Geometry: final body of the model. Coordinates: model frame, mm. A direction names the side the tool comes from. Give positions to 0.01 mm unless a question says otherwise; leave off trailing zeros. Write each loop counter-clockwise with the first axis right and the second up, starting at its lowest first coordinate (ties: lowest second). Pieces come first, ordered by that corner, then holes. Notation, with made-up numbers: M 29.5,65 L 72.5,65 A29 cw 72.5,91 Z; hole C -37,85.5 d11. An arc over 180 degrees is marked long. Use one line per item in the form item = value. Start each with the question number.
Item 1: Section query B-B on y = -25.5. Return loops of the section in (x, z).
Item 2: Access query for faces 1 (the flat face through (-27, -28.875, 12)), 2 (the flat face through (-41.999, -28, 12)). Directions: +Z, -Z, +X, -X, +Y, -Y. A direction counts if a zero-diameter tool reaches every point of the face in a straight line with its end or side. Return the directions, or none.
Item 3: Section query A-A on z = 10.75. Return loops of the section in (x, y), then the cut area to 3 significant figures.
Item 4: Contact query for flat-ended pins moving along their axis: P1, Ø2, axis at y = -27, z = 9, coming from the +X side; P2, Ø4.5, axis at x = -29, z = 10, coming from the +Y side; P3, Ø1, axis at x = -37.5, z = 7.5, coming from the -Y side (3 decimals). Output: stop coordinate, or through.
Item 5: Section query C-C on x = -30.5. Return loops of the section in (y, z).
Item 6: Material intervals for line 1 along X through (y, z) = (-26.75, 6.5); line 2 along Y through (x, z) = (-31.75, 10.75); line 3 along Y through (x, z) = (-25.25, 12), sorted ascending. Write a range as from..to.
from build123d import *

# Parameters (mm, degrees)
F1_DEPTH = 25


with BuildPart() as f1:
    # F0 (on Top) → F1 (new body)
    with BuildSketch(Plane.XY):
        Polygon((-32.0135473862, -18.9185493521), (-41.9985689223, -18.371425122), (-41.9985689223, -38.371425122), (-22.0037322274, -38.8258539341), (-22.9987681159, -28.8754819018), (-32.0135473862, -28.8754819018), align=None)
    extrude(amount=F1_DEPTH)


with BuildPart() as f1b:
    # F0 (on Top) → F1, piece 2 (new body)
    with BuildSketch(Plane.XY):
        Polygon((23.4582594037, -14.5173627138), (13.4582594037, -14.5173627138), (13.4582594037, -34.5173627138), (33.4582594037, -34.5173627138), (33.4582594037, -24.5173627138), (23.4582594037, -24.5173627138), align=None)
    extrude(amount=F1_DEPTH)


solid = f1.part
Answer sheet:
q1.outline = M -42,0 L -32.01,0 L -32.01,25 L -42,25 Z
q2.face_1 = +Z, -Z, +X, +Y
q2.face_2 = +Z, -Z, -X, +Y, -Y
q3.outline = M -42,-38.37 L -22,-38.83 L -23,-28.88 L -32.01,-28.88 L -32.01,-18.92 L -42,-18.37 Z
q3.area = 292 mm2
q4.P1 = -32.01
q4.P2 = -28.88
q4.P3 = -38.485
q5.outline = M -38.63,0 L -28.88,0 L -28.88,25 L -38.63,25 Z
q6.line_1 = -42..-32.01
q6.line_2 = -38.6..-28.88
q6.line_3 = -38.75..-28.88
